Can you work these out from the drawing? Everything is in mm from the part's minimum corner. A direction names the side the tool comes from. Round coordinates to 2 decimals unless told otherwise and drop trailing zeros. Loops run counter-clockwise (first coordinate to the right, second up) from the corner with the lowest first, then second, coordinate; pieces in that order, holes last. Notation, with made-up numbers: (49, 48.5) - (83, 48.5) arc R12 ccw to (83, 66.5) - close; hole circle Ø3 at (59.5, 89). An arc over 180 degrees is marked (long way). Put each result on its own line as item: value. Start each with the question number.
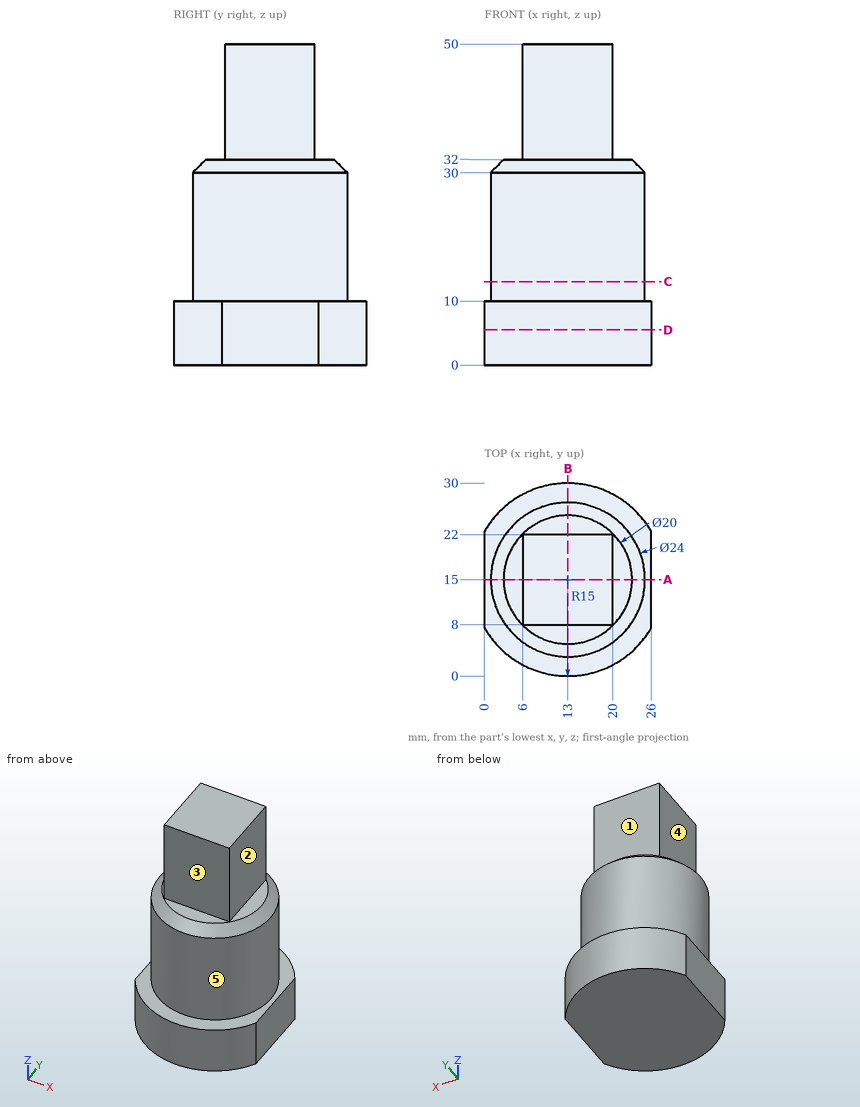
Item 1: Suppose I cut it at D-D, the plane z = 5.5. List the corners of the cut face in (x, y) for me.
Item 2: Will these pins go through, and if not, where does the flat tip stop? P1, Ø4, axis at x = 13, z = 45, coming from the -Y side; P2, Ø1, axis at x = 4, z = 34.5, coming from the -Y side; P3, Ø2, axis at y = 15.5, z = 25.5, coming from the +X side; P4, Ø11, axis at y = 16.5, z = 41.5, coming from the +X side.
Item 3: Suppose I cut it at C-C, the plane z = 13. List the corners of the cut face in (x, y) for me, then the cut area to 3 significant figures.
Item 4: Suppose I cut it at A-A, the plane y = 15. List the corners of the cut face in (x, z) for me, then the cut area to 3 significant figures.
Item 5: Suppose I cut it at B-B, the plane x = 13. List the corners of the cut face in (y, z) for me, then the cut area to 3 significant figures.
Item 6: I need wall thicknesses on line 1 (Y direction, x = 16.5, z = 33.5); line 2 (Y direction, x = 13.25, z = 14); line 3 (X direction, y = 15.5, z = 16.5). Which ranges of each line are inside material? Lowest first, please. Write a range as from..to.
Item 7: On a 3-axis mill with a long thin cutter (end or side, diameter ignored), from which of +Z, -Z, +X, -X, +Y, -Y can I reach the whole of each face in a straight line? I mean the marked faces 1, 2, 3, 4 and 5. Say none if no direction works.
Numbers:
1. outline: (0, 7.52) arc R15 ccw to (26, 7.52) - (26, 22.48) arc R15 ccw to (0, 22.48) - close
2. P1: y = 8
2. P2: through
2. P3: x = 25
2. P4: x = 20
3. outline: circle Ø24 at (13, 15)
3. area: 452 mm^2
4. outline: (0, 0) - (26, 0) - (26, 10) - (25, 10) - (25, 30) - (23, 32) - (20, 32) - (20, 50) - (6, 50) - (6, 32) - (3, 32) - (1, 30) - (1, 10) - (0, 10) - close
4. area: 1,040 mm^2
5. outline: (0, 0) - (30, 0) - (30, 10) - (27, 10) - (27, 30) - (25, 32) - (22, 32) - (22, 50) - (8, 50) - (8, 32) - (5, 32) - (3, 30) - (3, 10) - (0, 10) - close
5. area: 1,080 mm^2
6. line 1: 8..22
6. line 2: 3..27
6. line 3: 1.01..24.99
7. face 1: +Z, +X, -X, +Y
7. face 2: +Z, +X, +Y, -Y
7. face 3: +Z, +X, -X, -Y
7. face 4: +Z, -X, +Y, -Y
7. face 5: +Z
